Input: part model. Units: mm. Frame: model coordinates. Face numbers are marked on the shaded views. Coordinates: 2 decimals unless noted, no trailing zeros. Order: outer loops, then holes, each group sorted by start corner. A loop starts at its lowest first (then second) coordinate and runs counter-clockwise, first axis right, second up.
from build123d import *

# Parameters (mm, degrees)
SKETCH1_W                                       = 120
SKETCH1_H                                       = 70
SKETCH1_R                                       = 9.5
SKETCH1_R_2                                     = 2.5
BOSS_EXTRUDE1_DEPTH                             = 6
CSK_FOR_M3_FLAT_HEAD_MACHINE_SCREW1_D           = 3.2
CSK_FOR_M3_FLAT_HEAD_MACHINE_SCREW1_CSINK_D     = 6.3
CSK_FOR_M3_FLAT_HEAD_MACHINE_SCREW1_CSINK_ANGLE = 90


with BuildPart() as part:
    # Sketch1 → Boss-Extrude1 (new body)
    with BuildSketch(Plane(origin=(0, 0, 0), x_dir=(1, 0, 0), z_dir=(0, 1, 0))):
        Rectangle(SKETCH1_W, SKETCH1_H)
        Circle(SKETCH1_R, mode=Mode.SUBTRACT)
        with Locations((-17.5, 25)):
            Circle(SKETCH1_R_2, mode=Mode.SUBTRACT)
        with Locations((17.5, 25)):
            Circle(SKETCH1_R_2, mode=Mode.SUBTRACT)
        with Locations((17.5, -25)):
            Circle(SKETCH1_R_2, mode=Mode.SUBTRACT)
        with Locations((-17.5, -25)):
            Circle(SKETCH1_R_2, mode=Mode.SUBTRACT)
        with Locations((-50, 25)):
            Circle(SKETCH1_R_2, mode=Mode.SUBTRACT)
        with Locations((-50, -25)):
            Circle(SKETCH1_R_2, mode=Mode.SUBTRACT)
        with Locations((50, -25)):
            Circle(SKETCH1_R_2, mode=Mode.SUBTRACT)
        with Locations((50, 25)):
            Circle(SKETCH1_R_2, mode=Mode.SUBTRACT)
    extrude(amount=BOSS_EXTRUDE1_DEPTH)

    # CSK for M3 Flat Head Machine Screw1 (through all)
    with Locations(Plane(origin=(0, 0, 0), x_dir=(-1, 0, 0), z_dir=(0, -1, 0))):
        with Locations((-13, 0), (0, -13), (13, 0), (0, 13)):
            CounterSinkHole(CSK_FOR_M3_FLAT_HEAD_MACHINE_SCREW1_D / 2, CSK_FOR_M3_FLAT_HEAD_MACHINE_SCREW1_CSINK_D / 2, counter_sink_angle=CSK_FOR_M3_FLAT_HEAD_MACHINE_SCREW1_CSINK_ANGLE)


solid = part.part
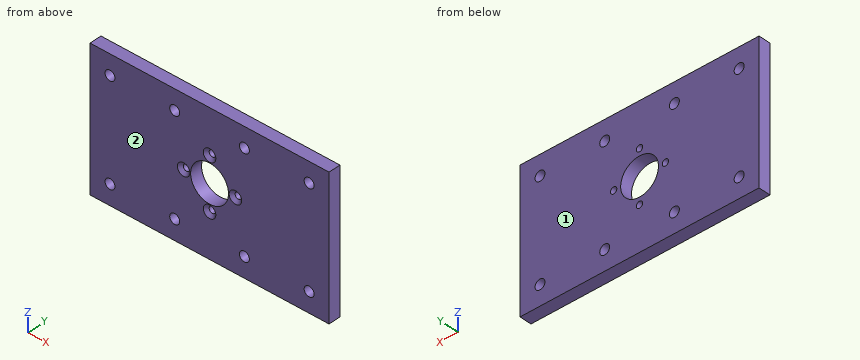
Item 1: Cut plane B-B on z = 13. Return loops of the section in (x, y).
Response values:
outline: (-60, 0) - (-3.15, 0) - (-1.6, 1.55) - (-1.6, 6) - (-60, 6) - close; (1.6, 1.55) - (3.15, 0) - (60, 0) - (60, 6) - (1.6, 6) - close
Item 2: Cut plane C-C on x = 0. Return loops of the section in (y, z), then the cut area to 3 significant figures.
Response values:
outline: (0, -35) - (6, -35) - (6, -14.6) - (1.55, -14.6) - (0, -16.15) - close; (0, -9.85) - (1.55, -11.4) - (6, -11.4) - (6, -9.5) - (0, -9.5) - close; (0, 9.5) - (6, 9.5) - (6, 11.4) - (1.55, 11.4) - (0, 9.85) - close; (0, 16.15) - (1.55, 14.6) - (6, 14.6) - (6, 35) - (0, 35) - close
area: 263 mm2
Item 3: Pin query (flat end, axial travel): pin 1 Ø6.5 at (x, z) = (-50, -25) entering from -Y. Return the tip coordinate at first contact, or that it passes through.
Response values:
pin 1: stops at y = 0
Item 4: Cut plane A-A on x = 13. Return loops of the section in (y, z), then the cut area to 3 significant figures.
Response values:
outline: (0, -35) - (6, -35) - (6, -1.6) - (1.55, -1.6) - (0, -3.15) - close; (0, 3.15) - (1.55, 1.6) - (6, 1.6) - (6, 35) - (0, 35) - close
area: 398 mm2
Item 5: Ray query, probe 1 along X at (y, z) = (1.45, 25); probe 2 along Z at (x, y) = (0, 3); probe 3 along X at (y, z) = (5.15, 1). Return the intervals inside material, ascending.
Response values:
probe 1: x = -60 to -52.5, -47.5 to -20, -15 to 15, 20 to 47.5, 52.5 to 60
probe 2: z = -35 to -14.6, -11.4 to -9.5, 9.5 to 11.4, 14.6 to 35
probe 3: x = -60 to -14.25, -11.75 to -9.45, 9.45 to 11.75, 14.25 to 60
Item 6: Cut plane D-D on z = 25. Return loops of the section in (x, y).
Response values:
outline: (-60, 0) - (-52.5, 0) - (-52.5, 6) - (-60, 6) - close; (-47.5, 0) - (-20, 0) - (-20, 6) - (-47.5, 6) - close; (-15, 0) - (15, 0) - (15, 6) - (-15, 6) - close; (20, 0) - (47.5, 0) - (47.5, 6) - (20, 6) - close; (52.5, 0) - (60, 0) - (60, 6) - (52.5, 6) - close
Item 7: Draft query along Y for the marked faces 1 and 2. Return one class per face: pulls with the +Y half, pulls with the -Y half, needs draft (parallel to the pull), parting line crosses it, or undercut.
Response values:
face 1: pulls with the +Y half
face 2: pulls with the -Y half
